```python
from build123d import *

# Parameters (mm, degrees)
F0_W            = 80
F0_H            = 60
F0_W_2          = 75
F0_H_2          = 55
F1_DEPTH        = 50
F0_R            = 1.55
F2_DEPTH        = 2.5
F3_W            = 10
F3_H            = 12
F3_R            = 1.55
F3_W_2          = 12
F3_H_2          = 10
F4_DEPTH        = 6
F5_R            = 2
F10_D           = 3.1
F10_CSINK_D     = 7.1
F10_CSINK_ANGLE = 82


with BuildPart() as f1:
    # F0 (on Front) → F1 (new body)
    with BuildSketch(Plane.XZ):
        Rectangle(F0_W, F0_H)
        Rectangle(F0_W_2, F0_H_2, mode=Mode.SUBTRACT)
    extrude(amount=-F1_DEPTH)

    # F0 (on Front) → F2 (join)
    with BuildSketch(Plane.XZ):
        Rectangle(F0_W_2, F0_H_2)
        with Locations((-0.25, -19)):
            Circle(F0_R, mode=Mode.SUBTRACT)
        with Locations((-0.25, 19)):
            Circle(F0_R, mode=Mode.SUBTRACT)
        Polygon((30.75, -9.5), (23.75, -14), (-23.75, -14), (-23.75, 14), (23.75, 14), (30.75, 9.5), align=None, mode=Mode.SUBTRACT)
    extrude(amount=-F2_DEPTH)

    # F3 (on face) → F4 (join)
    with BuildSketch(Plane(origin=(0, 50, 0), x_dir=(-1, 0, 0), z_dir=(0, 1, 0))):
        with Locations((45, 0)):
            Rectangle(F3_W, F3_H)
        with Locations((45, 0)):
            Circle(F3_R, mode=Mode.SUBTRACT)
        with Locations((3.022505, -35)):
            Rectangle(F3_W_2, F3_H_2)
        with Locations((3.022505, -35)):
            Circle(F3_R, mode=Mode.SUBTRACT)
        with Locations((-45, 0)):
            Rectangle(F3_W, F3_H)
        with Locations((-45, 0)):
            Circle(F3_R, mode=Mode.SUBTRACT)
        with Locations((3.022505, 35)):
            Rectangle(F3_W_2, F3_H_2)
        with Locations((3.022505, 35)):
            Circle(F3_R, mode=Mode.SUBTRACT)
    extrude(amount=-F4_DEPTH)

    # F5
    f5_edges = [f1.edges().sort_by_distance(p)[0] for p in [
        (40, 0, 0),
        (-40, 0, 0),
        (0, 0, 30),
        (0, 0, -30),
    ]]
    fillet(f5_edges, radius=F5_R)

    # F10 (through all)
    with Locations(Plane.XZ.offset(-44)):
        with Locations((-3.022505, -35), (-3.022505, 35), (-45, 0), (45, 0)):
            CounterSinkHole(F10_D / 2, F10_CSINK_D / 2, counter_sink_angle=F10_CSINK_ANGLE)


solid = f1.part
```
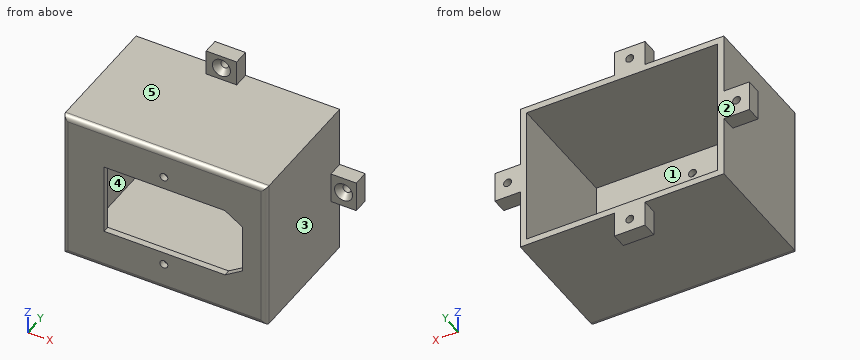
Verification items for the finished model (mm, model axes). Face numbers are marked on the shaded views. A direction names the side the tool comes from. Give positions to 0.01 mm unless a question says otherwise; leave off trailing zeros. Order: outer loops, then holes, each group sorted by start corner. A loop starts at its lowest first (then second) coordinate and runs counter-clockwise, first axis right, second up. Notation, with made-up numbers: (44, 79.25) - (80, 79.25) arc R31 cw to (80, 111.25) - close; hole circle Ø8 at (3, 46). An arc over 180 degrees is marked (long way). Answer as CSV lines item,"result". Start each with the question number.
Item 1: Section check A-A, the plane z = -19. Record the boundary of the cut face in (x, y), plus the area to 3 significant figures.
Item 2: Material ranges on L1, parallel to Z at x = -30, y = 42; L2, parallel to X at y = 49, z = 0; L3, parallel to Z at x = -45, y = 47.7, recorded low to high.
Item 3: Section check C-C, the plane x = -20.5. Record the boundary of the cut face in (y, z), plus the area to 3 significant figures.
Item 4: Mould release check, pull along X, two halves, no side actions. Record for the marked faces 3, 4 and 5: released by +X, released by -X, zero draft, split by the parting line, or undercut.
Item 5: Section check D-D, the plane z = 0. State how many separate pieces and enclosed holes the cut face has, plus the area to 3 significant figures.
Item 6: Gauge pin test, flat ends, axial feed: pin 1 (14.5 mm diameter, centred on x = -2.5, y = 24, fed in from -Z); pin 2 (2.5 mm diameter, centred on x = -45, z = 0, fed in from +Y); pin 3 (1 mm diameter, centred on y = 12, z = -21.5, fed in from -X); pin 4 (3 mm diameter, centred on y = 34.5, z = -2, fed in from +X). Record the tip position at first contact, or that the pin passes through.
Item 7: Section check B-B, the plane y = 38. Record the boundary of the cut face in (x, z).
Item 8: Access from +Z, -Z, +X, -X, +Y, -Y to the whole of each face (thin tool, end or side, straight path). Record for the marked faces 1 and 2.
Filled in:
1,outline,"(-40, 2) arc R2 ccw to (-38, 0) - (-1.8, 0) - (-1.8, 2.5) - (-37.5, 2.5) - (-37.5, 50) - (-40, 50) - close; (1.3, 0) - (38, 0) arc R2 ccw to (40, 2) - (40, 50) - (37.5, 50) - (37.5, 2.5) - (1.3, 2.5) - close"
1,area,"428 mm^2"
2,L1,"-30 to -27.5, 27.5 to 30"
2,L2,"-50 to -46.55, -43.45 to -37.5, 37.5 to 43.45, 46.55 to 50"
2,L3,"-6 to -1.55, 1.55 to 6"
3,outline,"(0, -28) arc R2 ccw to (2, -30) - (50, -30) - (50, -27.5) - (2.5, -27.5) - (2.5, -14) - (0, -14) - close; (0, 14) - (2.5, 14) - (2.5, 27.5) - (50, 27.5) - (50, 30) - (2, 30) arc R2 ccw to (0, 28) - close"
3,area,"316 mm^2"
4,face 3,"released by +X"
4,face 4,"undercut"
4,face 5,"zero draft"
5,separate pieces,"4"
5,enclosed holes,"0"
5,area,"373 mm^2"
6,pin 1,"z = -30"
6,pin 2,"through"
6,pin 3,"x = -40"
6,pin 4,"x = 40"
7,outline,"(-40, -30) - (40, -30) - (40, 30) - (-40, 30) - close; hole (-37.5, -27.5) - (37.5, -27.5) - (37.5, 27.5) - (-37.5, 27.5) - close"
8,face 1,"+Y"
8,face 2,"+Z, -Z, +X, -X, +Y"
